Autodesk Inventor part; units mm, degrees
ref_plane "Начальная плоскость" through (0, 0, 36) normal (0, 0, 1) x (1, 0, 0)
ref_plane "Конечная плоскость" through (0, 0, 171.172) normal (0, 0, 1) x (1, 0, 0)
ref_plane "РабПлоскость8" through (-343.772, 32.5, 171.172) normal (0, 0, 1) x (1, 0, 0)
ref_plane "Начальная плоскость" through (0, 0, 36) normal (0, 0, 1) x (1, 0, 0)
ref_plane "Конечная плоскость" through (0, 0, 171.172) normal (0, 0, 1) x (1, 0, 0)
sketch "Эскиз" plane through (0, 0, 0) normal (0, 0, 1) x (1, 0, 0)
  line L0 (36, -32.5) -> (0, -32.5)
  line L1 (36, -32.5) -> (36, -28.696)
  line L2 (33.6994, -26.2039) -> (9.9215, -24.3017)
  line L3 (4.4, -18.3208) -> (4.4, 18.3208)
  line L4 (33.6994, 26.2039) -> (9.9215, 24.3017)
  line L5 (36, 28.696) -> (36, 32.5)
  line L6 (0, 32.5) -> (36, 32.5)
  line L7 (0, -32.5) -> (0, 32.5)
  arc A0 (4.4, -18.3208) -> (9.9215, -24.3017) centre (10.4, -18.3208) ccw
  arc A1 (9.9215, 24.3017) -> (4.4, 18.3208) centre (10.4, 18.3208) ccw
  arc A2 (36, -28.696) -> (33.6994, -26.2039) centre (33.5, -28.696) ccw
  arc A3 (33.6994, 26.2039) -> (36, 28.696) centre (33.5, 28.696) ccw
  line L8 (0, 45.5) -> (0, -45.5) construction
  line L9 (-7.2974, 0) -> (43.7847, 0) construction
  point P0 (36, -26.388)
  point P1 (4.4, -23.86)
  point P2 (4.4, 23.86)
  point P3 (36, 26.388)
  dimension "d3" = 36
  dimension "d5" = 4.4
  dimension "d7" = 65
  dimension "d9" = 8.64
  dimension "d11" = 8.64
  dimension "d13" = 6.112
  dimension "d15" = 6.112
  dimension "d22" = 6
  dimension "d23" = 2.5
  dimension "d24" = 32.5
  dimension "d25" = 0
extrude "Тело" add sketch "Эскиз" along normal up to surface (135.172 mm away) from surface at 36
sketch "Sketch3" plane through (0, 0, 0) normal (0, 0, 1) x (1, 0, 0)
  line L0 (0, 0) -> (10, 0)
ref_plane "Work Plane7" through (0, 0, 0) normal (0, -1, 0) x (1, 0, 0)
sketch "Sketch4" plane through (0, 0, 0) normal (0, -1, 0) x (1, 0, 0)
  line L0 (-2, 36) -> (12, 36)
  line L1 (-2, 171.172) -> (12, 171.172)
  dimension "d29" = 135.172
ref_plane "РабПлоскость8" through (-343.772, 32.5, 171.172) normal (0, 0, 1) x (1, 0, 0)
split "Разделение1" plane through (-343.772, 32.5, 171.172) removes the side toward (0, 0, 1)
ref_plane "РабПлоскость9" through (-343.772, -32.5, 36) normal (0, 0, -1) x (-1, 0, 0)
split "Разделение2" plane through (-343.772, -32.5, 36) removes the side toward (0, 0, -1)
equation "\"d3\" = b"
equation "\"d7\" = ParH"
equation "\"d22\" = R"
equation "\"d23\" = R1"
equation "\"d24\" = 0.5 * d7"
equation "\"d16\" = G_L"
equation "\"R1\" = 2.5"
equation "\"R\" = 6"
equation "\"t1\" = 4.4"
equation "\"t2\" = 7.2"
equation "\"ParH\" = 65"
equation "\"b\" = 36"
equation "\"msp_x1\" = 0.04 * b"
equation "\"msp_x2\" = -0.08 * t1 + 0.04 * b"
equation "\"G_L\" = d29"
equation "\"ex\" = 0"
equation "\"G_OFFSET_START\" = -36"
equation "\"G_OFFSET_END\" = -36"
equation "\"d26\" = -G_OFFSET_START"
equation "\"d27\" = G_OFFSET_END + B_L"
equation "\"B_L\" = 207.172"
properties part number "Швеллер 6.5U-135,17 ГОСТ 8240-97" material "Сталь, мягкая"
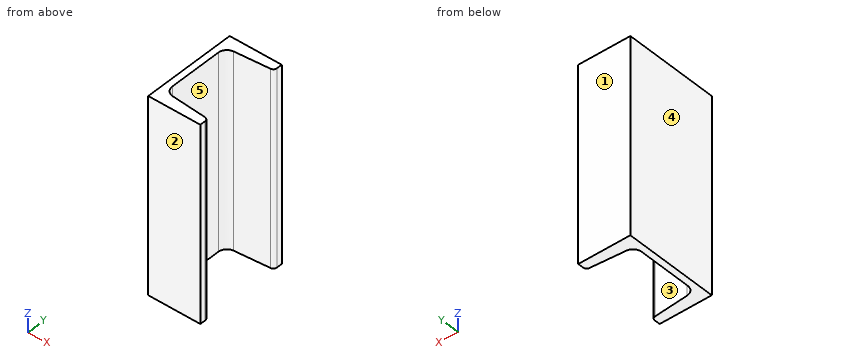
Can you work these out from the model? Positions are in its coordinate system, mm. Face numbers are marked on the shaded views. A direction names the side the tool comes from. Coordinates: 2 decimals unless noted, no trailing zeros. Write each loop counter-clockwise with the first axis right and the second up, starting at its lowest first coordinate (ties: lowest second). Pieces come first, ordered by that corner, then holes. Notation, with made-up numbers: M 5.5,60.5 L 23.5,60.5 A5 ccw 23.5,69.5 Z; hole C 29.5,13 d6. An arc over 180 degrees is marked long. Write item = value, one per line. Start each with the question number.
Q1. Thinking about a two-plate mould opening in Y: for the marked faces 1, 2 and 3, which applies, released by +Y, released by -Y, zero draft, split by the parting line, or undercut?
Q2. If we section it at C-C, the plane y = 4.5: Write out the boundary of the cut face in (x, z), then the cut area to 3 significant figures.
Q3. On a 3-axis mill with a long thin cutter (end or side, diameter ignored), from which of +Z, -Z, +X, -X, +Y, -Y can I reach the whole of each face in a straight line? I mean the marked faces 4 and 5. Say none if no direction works.
Q4. If we section it at A-A, the plane x = 17.5: Write out the boundary of the cut face in (y, z).
Q5. I'm going to push a flat-ended pin straight in: pin 1 (6 mm diameter, centred on y = -13, z = 150.5, fed in from +X). Where does the tip first touch, or does it pass through?
Q6. If I drill on L1, parallel to X at y = -1, z = 144; L2, parallel to Y at x = 31.5, z = 94; L3, parallel to Y at x = 26, z = 138.5, over which ranges is the centre line in solid material (lowest first)? Write a range as [from, to].
Q7. If we section it at D-D, the plane x = 6: Write out the boundary of the cut face in (y, z).
Q8. If we section it at B-B, the plane z = 106.5: Write out the boundary of the cut face in (x, y).
Check sheet entries:
q1.face_1 = released by +Y
q1.face_2 = released by -Y
q1.face_3 = undercut
q2.outline = M 0,36 L 4.4,36 L 4.4,171.17 L 0,171.17 Z
q2.area = 595 mm²
q3.face_4 = +Z, -Z, -X, +Y, -Y
q3.face_5 = +Z, -Z, +X
q4.outline = M -32.5,36 L -24.91,36 L -24.91,171.17 L -32.5,171.17 Z; M 24.91,36 L 32.5,36 L 32.5,171.17 L 24.91,171.17 Z
q5.pin_1 = 4.4
q6.L1 = [0, 4.4]
q6.L2 = [-32.5, -26.03], [26.03, 32.5]
q6.L3 = [-32.5, -25.59], [25.59, 32.5]
q7.outline = M -32.5,36 L -22.4,36 L -22.4,171.17 L -32.5,171.17 Z; M 22.4,36 L 32.5,36 L 32.5,171.17 L 22.4,171.17 Z
q8.outline = M 0,-32.5 L 36,-32.5 L 36,-28.7 A2.5 ccw 33.7,-26.2 L 9.92,-24.3 A6 cw 4.4,-18.32 L 4.4,18.32 A6 cw 9.92,24.3 L 33.7,26.2 A2.5 ccw 36,28.7 L 36,32.5 L 0,32.5 Z
